from build123d import *

# Parameters (mm, degrees)
SKETCH1_W                 = 38.1
SKETCH1_H                 = 50.8
BOSS_EXTRUDE1_DEPTH       = 19.05
SKETCH2_W                 = 19.05
SKETCH2_H                 = 50.8
CUT_EXTRUDE1_DEPTH        = 12.7
SKETCH3_W                 = 38.1
SKETCH3_H                 = 19.05
CUT_EXTRUDE2_DEPTH        = 12.7
F_1_4_CLEARANCE_HOLE1_D   = 6.7564
F_8_32_TAPPED_HOLE1_D     = 3.4544
F_8_32_TAPPED_HOLE1_DEPTH = 10.668
F_8_32_TAPPED_HOLE1_TIP   = 1.037806461


with BuildPart() as part:
    # Sketch1 → Boss-Extrude1 (new, symmetric)
    with BuildSketch(Plane.XY):
        Rectangle(SKETCH1_W, SKETCH1_H)
    extrude(amount=BOSS_EXTRUDE1_DEPTH, both=True)

    # Sketch2 → Cut-Extrude1 (cut)
    with BuildSketch(Plane(origin=(0, 0, -19.05), x_dir=(-1, 0, 0), z_dir=(0, 0, -1))):
        Rectangle(SKETCH2_W, SKETCH2_H)
    extrude(amount=-CUT_EXTRUDE1_DEPTH, mode=Mode.SUBTRACT)

    # Sketch3 → Cut-Extrude2 (cut)
    with BuildSketch(Plane.XY.offset(19.05)):
        with Locations((0, 9.525)):
            Rectangle(SKETCH3_W, SKETCH3_H)
    extrude(amount=-CUT_EXTRUDE2_DEPTH, mode=Mode.SUBTRACT)

    # 1/4 Clearance Hole1 (through all)
    with Locations(Plane.XY.offset(19.05)):
        with Locations((0, -15.875)):
            Hole(F_1_4_CLEARANCE_HOLE1_D / 2)

    # #8-32 Tapped Hole1
    with Locations(Plane.XY.offset(6.35)):
        with Locations((0, 9.525)):
            Hole(F_8_32_TAPPED_HOLE1_D / 2, depth=F_8_32_TAPPED_HOLE1_DEPTH)
            with Locations((0, 0, -(F_8_32_TAPPED_HOLE1_DEPTH + F_8_32_TAPPED_HOLE1_TIP / 2))):  # 118° drill point
                Cone(0, F_8_32_TAPPED_HOLE1_D / 2, F_8_32_TAPPED_HOLE1_TIP, mode=Mode.SUBTRACT)


solid = part.part
Read the model definition and answer for the solid it produces. Units are mm, in the model's axes. A direction names the side the tool comes from. Give positions to 0.01 mm unless a question says otherwise; leave off trailing zeros. Write each loop counter-clockwise with the first axis right and the second up, starting at its lowest first coordinate (ties: lowest second). Pieces come first, ordered by that corner, then holes. Notation, with made-up numbers: (18, -8) - (33, -8) arc R31 cw to (33, 21) - close; hole circle Ø5 at (-2.5, 31.25). An arc over 180 degrees is marked (long way). Use CSV: the item, a comma, the result in double quotes. Start each with the question number.
(1) Find section D-D (z = 8). Give the vertices of the cut face in (x, y) (3 decimals), plus the area to 3 significant figures.
(2) Find section B-B (x = 15). Give the vertices of the cut face in (y, z).
(3) Consider line 1 along Y through (x, z) = (0, 2); line 2 along Y through (x, z) = (0, 13); line 3 along X through (y, z) = (-6, -10) (3 decimals). Determine where each line is inside the solid, lowest interval first.
(4) Find section A-A (z = -10). Give the vertices of the cut face in (x, y) (3 decimals).
(5) Find section C-C (y = 21.5). Give the vertices of the cut face in (x, z) (3 decimals), plus the area to 3 significant figures.
(6) For faces 1 (the flat face through (0, 12, 6.35)), 2 (the flat face through (9.525, 0, -13)), 3 (the cylindrical face through (0.22, 11.24, 0.94)), 4 (the flat face through (0, 22, 19.05)), 5 (the flat face through (0, 25.4, 5)), determine the directions among +Z, -Z, +X, -X, +Y, -Y from which every point of the face is accessible in a straight line to the end or side of a thin tool.
(7) Determine the mould class of faces 6 (the flat face through (-19.05, 0, 0)), 7 (the flat face through (0, 0, -6.35)), 8 (the flat face through (0, 0, 13)) for opening direction X: +X half, -X half, draft (parallel to the pull), parting line (faces both ways), or undercut.
(8) Given P1, Ø3, axis at x = 11, y = 18.5, coming from the +Z side; P2, Ø4, axis at x = 0, y = 9.525, coming from the -Z side; P3, Ø6, axis at x = 0, y = -15.875, coming from the -Z side, each flat-ended and moving along its own axis, determine where each tip first touches the part or whether it passes through.
Findings below:
1,outline,"(-19.05, -25.4) - (19.05, -25.4) - (19.05, 0) - (-19.05, 0) - close; (-19.05, 19.05) - (19.05, 19.05) - (19.05, 25.4) - (-19.05, 25.4) - close; hole circle Ø6.756 at (0, -15.875)"
1,area,"1,170 mm2"
2,outline,"(-25.4, -19.05) - (25.4, -19.05) - (25.4, 19.05) - (19.05, 19.05) - (19.05, 6.35) - (0, 6.35) - (0, 19.05) - (-25.4, 19.05) - close"
3,line 1,"-25.4 to -19.25, -12.5 to 7.8, 11.25 to 25.4"
3,line 2,"-25.4 to -19.25, -12.5 to 0, 19.05 to 25.4"
3,line 3,"-19.05 to -9.525, 9.525 to 19.05"
4,outline,"(-19.05, -25.4) - (-9.525, -25.4) - (-9.525, 25.4) - (-19.05, 25.4) - close; (9.525, -25.4) - (19.05, -25.4) - (19.05, 25.4) - (9.525, 25.4) - close"
5,outline,"(-19.05, -19.05) - (-9.525, -19.05) - (-9.525, -6.35) - (9.525, -6.35) - (9.525, -19.05) - (19.05, -19.05) - (19.05, 19.05) - (-19.05, 19.05) - close"
5,area,"1,210 mm2"
6,face 1,"+Z, +X, -X"
6,face 2,"-Z, +Y, -Y"
6,face 3,"+Z"
6,face 4,"+Z, +X, -X, +Y, -Y"
6,face 5,"+Z, -Z, +X, -X, +Y"
7,face 6,"-X half"
7,face 7,"undercut"
7,face 8,"draft"
8,P1,"z = 19.05"
8,P2,"z = -6.35"
8,P3,"through"
